Can you work these out from the model? Positions are in its coordinate system, mm. Face numbers are marked on the shaded views. A direction names the side the tool comes from. Round coordinates to 2 decimals unless told otherwise and drop trailing zeros. Order: outer loops, then holes, each group sorted by start corner. A loop starts at its lowest first (then second) coordinate and runs counter-clockwise, first axis right, second up. Notation, with made-up numbers: (-13.5, 89.5) -> (18.5, 89.5) arc R13 cw to (18.5, 113.5) -> close; hole circle Ø4 at (-28, 86.5). An arc over 180 degrees is marked (long way). Use a Markdown table: item, result. Add a question column.
Q1. If we section it at C-C on z = 60.5: List the corners of the cut face in (x, y) for me.
Q2. I need wall thicknesses on line 1 along X through (y, z) = (-45, 4); line 2 along Y through (x, z) = (10.5, 37); line 3 along Z through (x, y) = (114.5, 0). Which ranges of each line are inside material? Lowest first, please. Write a range as [from, to].
Q3. We'd pull the mould along X, two halves only. Please class the marked faces 1, 2 and 3: +X half, -X half, draft (parallel to the pull), parting line (faces both ways), or undercut.
Q4. If we section it at A-A on y = 37: List the corners of the cut face in (x, z) for me.
Q5. I'm going to push a flat-ended pin straight in: pin 1 Ø9 at (x, y) = (23.5, -69.5) entering from +Z. Where does the tip first touch, or does it pass through?
Q6. If we section it at D-D on y = 0: List the corners of the cut face in (x, z) for me, plus the area to 3 significant figures.
Q7. If we section it at B-B on x = 20.5: List the corners of the cut face in (y, z) for me.
Q8. For the marked faces 4 and 5, which set-ups out of +Z, -Z, +X, -X, +Y, -Y let a thin tool reach every point of the face, with its end or its side?
```python
from build123d import *

# Parameters (mm, degrees)
F0_W     = 236.464172
F0_H     = 153.010204
F1_DEPTH = 89.154
F2_W     = 219.41261
F2_H     = 130.49218
F3_DEPTH = 170.434
F4_W     = 99.966138
F4_H     = 51.93973
F5_DEPTH = 169.926
F6_R     = 15.346297
F7_DEPTH = 355.854


with BuildPart() as f1:
    # F0 (on Top) → F1 (new body)
    with BuildSketch(Plane.XY):
        Rectangle(F0_W, F0_H)
    extrude(amount=F1_DEPTH)

    # F2 (on face) → F3 (cut)
    with BuildSketch(Plane.XY.offset(89.154)):
        Rectangle(F2_W, F2_H)
    extrude(amount=-F3_DEPTH, mode=Mode.SUBTRACT)

    # F4 (on face) → F5 (cut)
    with BuildSketch(Plane.XZ.offset(76.505102)):
        with Locations((0, 89.154)):
            Rectangle(F4_W, F4_H)
    extrude(amount=-F5_DEPTH, mode=Mode.SUBTRACT)

    # F6 (on face) → F7 (cut)
    with BuildSketch(Plane.YZ.offset(118.232086)):
        with Locations((0, 42.181458)):
            Circle(F6_R)
    extrude(amount=-F7_DEPTH, mode=Mode.SUBTRACT)


solid = f1.part
```
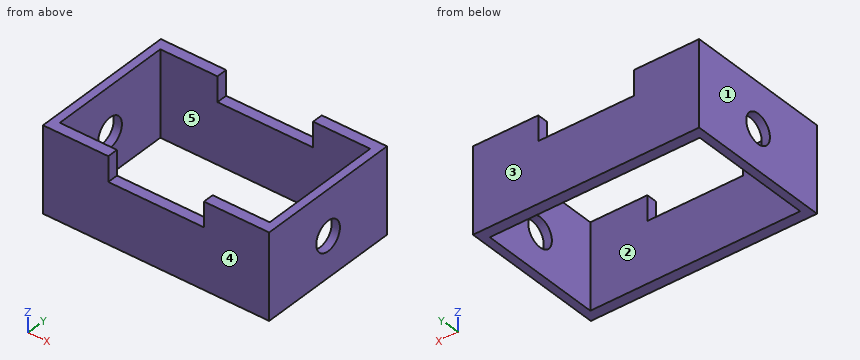
Answer below:
| question | item | result |
|---|---|---|
| 1 | outline | (-118.23, -76.51) -> (118.23, -76.51) -> (118.23, 76.51) -> (-118.23, 76.51) -> close; hole (-109.71, -65.25) -> (109.71, -65.25) -> (109.71, 65.25) -> (-109.71, 65.25) -> close |
| 2 | line 1 | [-118.23, -109.71], [109.71, 118.23] |
| 2 | line 2 | [-76.51, -65.25], [65.25, 76.51] |
| 2 | line 3 | [0, 26.84], [57.53, 89.15] |
| 3 | face 1 | -X half |
| 3 | face 2 | undercut |
| 3 | face 3 | draft |
| 4 | outline | (-118.23, 0) -> (-109.71, 0) -> (-109.71, 89.15) -> (-118.23, 89.15) -> close; (109.71, 0) -> (118.23, 0) -> (118.23, 89.15) -> (109.71, 89.15) -> close |
| 5 | pin 1 | z = 63.18 |
| 6 | outline | (-118.23, 0) -> (-109.71, 0) -> (-109.71, 26.84) -> (-118.23, 26.84) -> close; (-118.23, 57.53) -> (-109.71, 57.53) -> (-109.71, 89.15) -> (-118.23, 89.15) -> close; (109.71, 0) -> (118.23, 0) -> (118.23, 26.84) -> (109.71, 26.84) -> close; (109.71, 57.53) -> (118.23, 57.53) -> (118.23, 89.15) -> (109.71, 89.15) -> close |
| 6 | area | 997 mm² |
| 7 | outline | (-76.51, 0) -> (-65.25, 0) -> (-65.25, 63.18) -> (-76.51, 63.18) -> close; (65.25, 0) -> (76.51, 0) -> (76.51, 63.18) -> (65.25, 63.18) -> close |
| 8 | face 4 | +Z, -Z, +X, -X, -Y |
| 8 | face 5 | +Z, -Z |
